```python
from build123d import *

# Parameters (mm, degrees)
F1_DEPTH = 12.7
F2_W     = 25.4
F2_H     = 25.4
F3_DEPTH = 19.05
F5_DEPTH = 25.4


with BuildPart() as f1:
    # F0 (on Top) → F1 (new body)
    with BuildSketch(Plane.XY):
        with BuildLine():
            Line((-34.4024921656, 12.6939360307), (-35.190372549, 12.6938412482))
            ThreePointArc((-35.190372549, 12.6938412482), (-47.493365494, -0.1977576135), (-34.7949052753, -12.7))
            ThreePointArc((-34.7949052753, -12.7), (-25.8146491543, -8.9802561211), (-22.0949052753, 0))
            ThreePointArc((-22.0949052753, 0), (-25.6769656371, 8.840428539), (-34.4024921656, 12.6939360307))
        make_face()
        with BuildLine():
            ThreePointArc((-34.4024921656, 12.6939360307), (-34.7964330925, 12.6999999081), (-35.190372549, 12.6938412482))
            Line((-35.190372549, 12.6938412482), (-34.4024921656, 12.6939360307))
        make_face()
        with BuildLine():
            ThreePointArc((-22.0949052753, 0), (-25.8146491543, -8.9802561211), (-34.7949052753, -12.7))
            Line((-34.7949052753, -12.7), (16.0050947247, -12.7))
            ThreePointArc((16.0050947247, -12.7), (3.3050947477, -0.0007639086), (16.0035669075, 12.6999999081))
            Line((16.0035669075, 12.6999999081), (-34.4024921656, 12.6939360307))
            ThreePointArc((-34.4024921656, 12.6939360307), (-25.6769656371, 8.840428539), (-22.0949052753, 0))
        make_face()
        with BuildLine():
            ThreePointArc((16.0035669075, 12.6999999081), (3.3050947477, -0.0007639086), (16.0050947247, -12.7))
            ThreePointArc((16.0050947247, -12.7), (24.9853508457, -8.9802561211), (28.7050947247, 0))
            ThreePointArc((28.7050947247, 0), (24.9848106646, 8.9807962698), (16.0035669075, 12.6999999081))
        make_face()
    extrude(amount=F1_DEPTH)

    # F2 (on Top) → F3 (join)
    with BuildSketch(Plane.XY):
        with Locations((-9.3933891925, -0.0239079818)):
            Rectangle(F2_W, F2_H)
    extrude(amount=F3_DEPTH)

    # F4 (on face) → F5 (join)
    with BuildSketch(Plane.YZ.offset(3.3066108075)):
        with BuildLine():
            Line((-12.7239079818, 19.05), (12.6760920182, 19.05))
            ThreePointArc((12.6760920182, 19.05), (-0.0239079818, 31.75), (-12.7239079818, 19.05))
        make_face()
    extrude(amount=-F5_DEPTH)


solid = f1.part
```
Check sheet for the modelled part. Datum: model origin and axes. Units: mm. Give positions to 0.01 mm unless a question says otherwise; leave off trailing zeros. Order: outer loops, then holes, each group sorted by start corner. A loop starts at its lowest first (then second) coordinate and runs counter-clockwise, first axis right, second up. Notation, with made-up numbers: (39.25, 6.5) -> (71.25, 6.5) arc R36 ccw to (71.25, 44.5) -> close; hole circle Ø11 at (60.25, 75). An arc over 180 degrees is marked (long way). Return JSON: item names as keys, results as strings.
1. Material ranges on probe 1 along X at (y, z) = (4.25, 16); probe 2 along Z at (x, y) = (21.5, -4); probe 3 along Y at (x, z) = (-16, 7), recorded low to high. Write a range as [from, to].
From the geometry:
{"probe 1": "[-22.09, 3.31]", "probe 2": "[0, 12.7]", "probe 3": "[-12.72, 12.7]"}
2. Cross-section at A-A, the plane y = 1.5. Record the cut outline in (x, z), plus the area to 3 significant figures.
From the geometry:
{"outline": "(-47.41, 0) -> (28.62, 0) -> (28.62, 12.7) -> (3.31, 12.7) -> (3.31, 31.66) -> (-22.09, 31.66) -> (-22.09, 12.7) -> (-47.41, 12.7) -> close", "area": "1,450 mm^2"}
3. Cross-section at B-B, the plane z = 13.5. Record the cut outline in (x, y), plus the area to 3 significant figures.
From the geometry:
{"outline": "(-22.09, -12.72) -> (3.31, -12.72) -> (3.31, 12.68) -> (-22.09, 12.68) -> close", "area": "645 mm^2"}
4. Go/stop test with flat-tipped pins: P1, Ø8, axis at y = -0.5, z = 26, coming from the -X side; P2, Ø10, axis at x = -21.5, z = 28, coming from the +Y side; P3, Ø6, axis at y = 0.5, z = 5, coming from the -X side; P4, Ø8, axis at x = 9, z = 26.5, coming from the +Y side. Record where each tip stops, or that it passes through.
From the geometry:
{"P1": "x = -22.09", "P2": "y = 12.05", "P3": "x = -47.49", "P4": "through"}
5. Cross-section at D-D, the plane y = 10.25. Record the cut outline in (x, z).
From the geometry:
{"outline": "(-42.29, 0) -> (23.5, 0) -> (23.5, 12.7) -> (3.31, 12.7) -> (3.31, 26.52) -> (-22.09, 26.52) -> (-22.09, 12.7) -> (-42.29, 12.7) -> close"}
